Build history of the part. All positions in model axes, mm. A direction names the side the tool comes from. Coordinates: 2 decimals unless noted, no trailing zeros. Order: outer loops, then holes, each group sorted by start corner. A loop starts at its lowest first (then second) coordinate and runs counter-clockwise, first axis right, second up. Notation, with made-up numbers: (65.5, 34) - (89.5, 34) arc R30 ccw to (89.5, 58) - close; hole circle Ø2 at (-11, 30). An arc over 180 degrees is marked (long way). Write each question's results on one line, items separated by ' | '.
from build123d import *

# Parameters (mm, degrees)
BOSS_EXTRUDE1_DEPTH = 1.5
BOSS_EXTRUDE2_DEPTH = 20
LPATTERN1_COUNT     = 2
LPATTERN1_PITCH     = 40
SKETCH4_R           = 2.5
CUT_EXTRUDE1_DEPTH  = 5.124819455
CHAMFER1_SIZE       = 0.5


with BuildPart() as part:
    # Sketch1 → Boss-Extrude1 (new body)
    with BuildSketch(Plane(origin=(0, 0, 0), x_dir=(1, 0, 0), z_dir=(0, 1, 0))):
        with BuildLine():
            Line((40, -17.5), (-40, -17.5))
            Line((-40, -17.5), (-40, 12.5))
            ThreePointArc((-40, 12.5), (-38.535533906, 16.035533906), (-35, 17.5))
            Line((-35, 17.5), (35, 17.5))
            ThreePointArc((35, 17.5), (38.535533906, 16.035533906), (40, 12.5))
            Line((40, 12.5), (40, -17.5))
        make_face()
    extrude(amount=BOSS_EXTRUDE1_DEPTH)

    # Sketch3 → Boss-Extrude2 (add)
    with BuildSketch(Plane(origin=(40, 0, 0), x_dir=(0, 0, -1), z_dir=(1, 0, 0))):
        with BuildLine():
            Line((-19.385927186, 2.712688903), (-17.728294567, 2.712688903))
            ThreePointArc((-17.728294567, 2.712688903), (-25.49630848, 1.493271308), (-17.813805195, -0.182486041))
            ThreePointArc((-17.813805195, -0.182486041), (-17.700741006, -0.047620698), (-17.531495251, 0.000629131))
            Line((-17.531495251, 0.000629131), (-17.5, 0))
            Line((-17.5, 0), (-17.5, 1.5))
            Line((-17.5, 1.5), (-18.703537452, 1.5))
            ThreePointArc((-18.703537452, 1.5), (-18.908926347, 1.418667331), (-19.002949729, 1.218769344))
            ThreePointArc((-19.002949729, 1.218769344), (-23.919742449, 0.754362088), (-19.385927186, 2.712688903))
        make_face()
    boss_extrude2 = extrude(amount=-BOSS_EXTRUDE2_DEPTH)

    # LPattern1: Boss-Extrude2 ×2
    with Locations(*[(-i * LPATTERN1_PITCH, 0, 0) for i in range(1, LPATTERN1_COUNT)]):
        add(boss_extrude2)

    # Sketch4 → Cut-Extrude1 (cut, through all)
    with BuildSketch(Plane(origin=(0, 1.5, 0), x_dir=(1, 0, 0), z_dir=(0, 1, 0))):
        with Locations((0, 7.5)):
            Circle(SKETCH4_R)
        with Locations((-26, -5.5)):
            Circle(SKETCH4_R)
        with Locations((26, -5.5)):
            Circle(SKETCH4_R)
    extrude(amount=-CUT_EXTRUDE1_DEPTH, mode=Mode.SUBTRACT)

    # Chamfer1
    chamfer1_edges = [part.edges().sort_by_distance(p)[0] for p in [
        (-2.5, 1.5, -7.5),
        (-28.5, 1.5, 5.5),
        (23.5, 1.5, 5.5),
    ]]
    chamfer(chamfer1_edges, length=CHAMFER1_SIZE)


solid = part.part
1. Probe line 1 (X direction, y = 0.5, z = 5.5); line 2 (X direction, y = -0.75, z = 23); line 3 (X direction, y = 0.7, z = -7.5). List the from-to ranges inside material, lowest first.
Solved:
line 1: x = -40 to -28.5, -23.5 to 23.5, 28.5 to 40 | line 2: x = -20 to 0, 20 to 40 | line 3: x = -40 to -2.5, 2.5 to 40
2. Band-saw the part on B-B on z = 5.5. Give the cut face in (x, y).
Solved:
outline: (-40, 0) - (-28.5, 0) - (-28.5, 1) - (-29, 1.5) - (-40, 1.5) - close; (-23.5, 0) - (23.5, 0) - (23.5, 1) - (23, 1.5) - (-23, 1.5) - (-23.5, 1) - close; (28.5, 0) - (40, 0) - (40, 1.5) - (29, 1.5) - (28.5, 1) - close
3. Band-saw the part on D-D on z = -3. Give the cut face in (x, y), then the cut area to 3 significant figures.
Solved:
outline: (-40, 0) - (40, 0) - (40, 1.5) - (-40, 1.5) - close | area: 120 mm2
4. Two-plate mould, pull along Z, no slides. Class faces 4 (the face through (-10, 2.713, 19)), 5 (the face through (-9.86, 1.65, 25.49)), 6 (the face through (-9.86, 0.659, 23.893)): +Z half, -Z half, draft (parallel to the pull), parting line (faces both ways), or undercut.
Solved:
face 4: draft | face 5: parting line | face 6: undercut
5. Band-saw the part on A-A on x = -26. Give the cut face in (y, z).
Solved:
outline: (0, -17.5) - (1.5, -17.5) - (1.5, 2.5) - (1, 3) - (0, 3) - close; (0, 8) - (1, 8) - (1.5, 8.5) - (1.5, 17.5) - (0, 17.5) - close
6. Drop flat-ended pins along their axis: pin 1 Ø1.8 at (x, z) = (-15, 18.5) entering from -Y; pin 2 Ø2 at (x, z) = (-24, -4) entering from -Y; pin 3 Ø0.5 at (x, z) = (35, 19) entering from -Y; pin 4 Ø3 at (y, z) = (1.38, 21.5) entering from -X. Give the stop position or say it passes through.
Solved:
pin 1: stops at y = -2.03 | pin 2: stops at y = 0 | pin 3: stops at y = -1.93 | pin 4: passes through
7. Tool access for faces 1 (the face through (1, 0, 0)), 2 (the face through (0, -1.2, 22.4)), 3 (the face through (38.5, 0.74, -16.07)): list every direction of +Z, -Z, +X, -X, +Y, -Y with a clear straight run to the whole face (end or side of a thin tool).
Solved:
face 1: -Z, +X, -X, -Y | face 2: +Z, +Y, -Y | face 3: -Z, +X, +Y, -Y
